Geometry check sheet. Reference: the model listing, model coordinates, mm. Face numbers are marked on the shaded views. Coordinates: 2 decimals unless noted, no trailing zeros. Order: outer loops, then holes, each group sorted by start corner. A loop starts at its lowest first (then second) coordinate and runs counter-clockwise, first axis right, second up. Notation, with made-up numbers: (55, 87) - (60, 87) arc R6 ccw to (60, 95) - close; hole circle Ø3 at (54, 13.5). An arc over 180 degrees is marked (long way). Use CSV: the item, a comma, the result in double quotes. Start each with the question number.
1) Thickness scan on probe 1 along Y at (x, z) = (0, -35.25) (3 decimals); probe 2 along X at (y, z) = (-9, -22); probe 3 along X at (y, z) = (-5, -22.5). Record the ranges inside material, lowest first. Write a range as [from, to].
2) Sectioned sample at B-B, the plane z = -29. Record the cut outline in (x, y).
3) Draft check along X on the marked faces 1, 2 and 3. Enter one of: released by +X, released by -X, zero draft, split by the parting line, or undercut.
4) Sectioned sample at A-A, the plane x = 0. Record the cut outline in (y, z) (1 decimal).
5) Depth check by flat-ended pin: P1, Ø4, axis at y = -3, z = -4, coming from the +X side; P2, Ø2, axis at x = 16, y = -10.5, coming from the +Z side; P3, Ø1.9, axis at x = -31, y = -9, coming from the +Z side. Enter the tip coordinate at first touch or a pass-through.
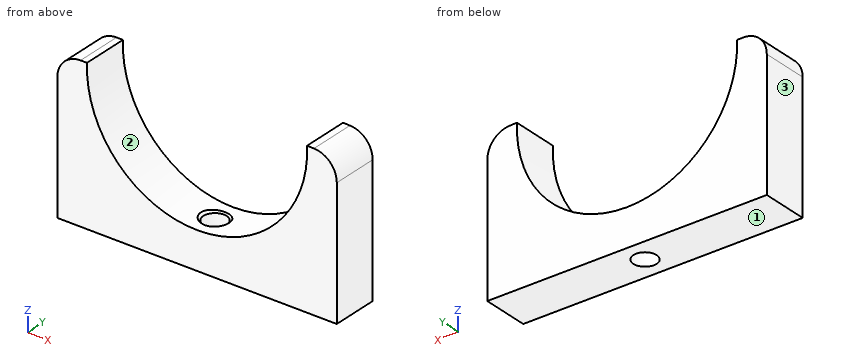
from build123d import *

# Parameters (mm, degrees)
F1_DEPTH    = 12.7
F3_R        = 4.7625
F4_DEPTH    = 6.35
F5_R        = 3.175
F6_DEPTH    = 12.7
F7_S5_R     = 30.0250138604
F7_T6_DEPTH = 8
F7_S7_R     = 3.175
F7_T8_DEPTH = 8
F8_R        = 6.35


# Not quite as in the source:
# - a fillet or chamfer that OpenCascade refuses, or shapes differently, is made with other operations: its cross-section is extruded or revolved along the edge and cut away or added


with BuildPart() as f1:
    # F0 (on Front) → F1 (new body)
    with BuildSketch(Plane.XZ):
        with BuildLine():
            Line((-38.1, 0), (-38.1, -41.275))
            Line((-38.1, -41.275), (38.1, -41.275))
            Line((38.1, -41.275), (38.1, 0))
            Line((38.1, 0), (30.0016984668, 0.169987541))
            ThreePointArc((30.0016984668, 0.169987541), (0.0893604764, -31.1423259445), (-29.9999146, 0))
            Line((-29.9999146, 0), (-38.1, 0))
        make_face()
    extrude(amount=F1_DEPTH)

    # F3 (on offset) → F4 (cut)
    with BuildSketch(Plane.XY.offset(-25.4)):
        with Locations((0, -6.35)):
            Circle(F3_R)
    extrude(amount=-F4_DEPTH, mode=Mode.SUBTRACT)

    # F5 (on face) → F6 (cut)
    with BuildSketch(Plane.XY.offset(-31.75)):
        with Locations((0, -6.35)):
            Circle(F5_R)
    extrude(amount=-F6_DEPTH, mode=Mode.SUBTRACT)

    # F7: chamfer of 1.778 on 1 edges, made by hand


with BuildPart() as f7_tool2:
    # F7_s3 → F7_t4 (revolve)
    with BuildSketch(Plane.XZ.offset(6.35)):
        Polygon((4.7625, -29.972), (2.9845, -31.75), (4.7625, -31.75), align=None)
    revolve(axis=Axis((0, -6.35, -31.75), (0, 0, 1)))

    # F7_s5 → F7_t6 (cut, symmetric)
    with BuildSketch(Plane.XZ.offset(6.3)):
        with Locations((0.0042984668, -1.1174325763)):
            Circle(F7_S5_R)
    extrude(amount=F7_T6_DEPTH, both=True, mode=Mode.SUBTRACT)

    # F7_s7 → F7_t8 (cut, symmetric)
    with BuildSketch(Plane.XY.offset(-30.9)):
        with Locations((0, -6.35)):
            Circle(F7_S7_R)
    extrude(amount=F7_T8_DEPTH, both=True, mode=Mode.SUBTRACT)


with BuildPart() as f1_1:
    add(f1.part)

    # F7_t1: union F7_tool2
    add(f7_tool2.part)

    # F8
    f8_edges = [f1_1.edges().sort_by_distance(p)[0] for p in [
        (-38.1, -6.35, 0),
        (38.1, -6.35, 0),
    ]]
    fillet(f8_edges, radius=F8_R)


solid = f1_1.part
Evaluation:
1,probe 1,"[-12.7, -9.525], [-3.175, 0]"
1,probe 2,"[-38.1, -21.57], [21.58, 38.1]"
1,probe 3,"[-38.1, -21.07], [21.08, 38.1]"
2,outline,"(-38.1, -12.7) - (-11.13, -12.7) - (-11.13, 0) - (-38.1, 0) - close; (11.14, -12.7) - (38.1, -12.7) - (38.1, 0) - (11.14, 0) - close"
3,face 1,"zero draft"
3,face 2,"undercut"
3,face 3,"released by -X"
4,outline,"(-12.7, -41.3) - (-9.5, -41.3) - (-9.5, -31.6) - (-9.9, -31.1) - (-12.7, -31.1) - close; (-3.2, -41.3) - (0, -41.3) - (0, -31.1) - (-2.8, -31.1) - (-3.2, -31.6) - close"
5,P1,"x = 38.1"
5,P2,"z = -25.87"
5,P3,"z = 0"
